```python
from build123d import *

# Parameters (mm, degrees)
BOSS_EXTRUDE1_DEPTH      = 355.6
BOSS_EXTRUDE1_DEPTH_BACK = 254
SKETCH1_R                = 66.04
FILLET1_R                = 12.7
SKETCH3_R                = 12.7
CUT_EXTRUDE1_DEPTH       = 25.4
CHAMFER1_SIZE            = 1.27
FILLET2_R                = 2.54
BOSS_EXTRUDE2_DEPTH      = 600
BOSS_EXTRUDE2_DEPTH_BACK = 583.65
SKETCH4_R                = 120
FILLET3_R                = 20
FILLET4_R                = 90


# Read off the part's stored shape, not the designer's step: Shell1
with BuildPart() as part:
    # Sketch1 → Boss-Extrude1 (new, two sides: drawn at the far end of the back side and taken through both)
    with BuildSketch(Plane.XY.offset(-BOSS_EXTRUDE1_DEPTH_BACK)):
        Circle(SKETCH1_R)
    extrude(amount=BOSS_EXTRUDE1_DEPTH + BOSS_EXTRUDE1_DEPTH_BACK)

    # Sketch2 → Cut-Revolve1 (revolve, cut)
    with BuildSketch(Plane(origin=(0, 0, 0), x_dir=(0, 0, -1), z_dir=(1, 0, 0)), mode=Mode.PRIVATE) as cut_revolve1_sk:
        with BuildLine():
            Line((-355.6, 19.05), (-330.2, 19.05))
            ThreePointArc((-330.2, 19.05), (-306.35774098, 53.006337357), (-266.967262435, 66.04))
            Line((-266.967262435, 66.04), (-355.6, 66.04))
            Line((-355.6, 66.04), (-355.6, 19.05))
        make_face()
    revolve(cut_revolve1_sk.sketch.rotate(Axis((0, 0, 355.6), (0, 0, -1)), 90), axis=Axis((0, 0, 355.6), (0, 0, -1)), mode=Mode.SUBTRACT)

    # Fillet1
    fillet1_edges = [part.edges().sort_by_distance(p)[0] for p in [
        (-66.04, 0, -254),
    ]]
    fillet(fillet1_edges, radius=FILLET1_R)

    # Sketch3 → Cut-Extrude1 (cut)
    with BuildSketch(Plane.XY.offset(355.6)):
        Circle(SKETCH3_R)
    extrude(amount=-CUT_EXTRUDE1_DEPTH, mode=Mode.SUBTRACT)

    # Shell1 outline → Shell1 (revolve, cut)
    with BuildSketch(Plane.XZ):
        with BuildLine():
            Line((0, -247.65), (53.34, -247.65))
            ThreePointArc((53.34, -247.65), (57.830128061, -245.790128061), (59.69, -241.3))
            Line((59.69, -241.3), (59.69, 266.967262375))
            ThreePointArc((59.69, 266.967262375), (46.480959005, 304.416114887), (12.699999942, 325.290551964))
            Line((12.699999942, 325.290551964), (12.7, 330.2))
            Line((12.7, 330.2), (0, 330.2))
            Line((0, 330.2), (0, -247.65))
        make_face()
    revolve(axis=Axis((0, 0, 0), (0, 0, 1)), mode=Mode.SUBTRACT)

    # Chamfer1
    chamfer1_edges = [part.edges().sort_by_distance(p)[0] for p in [
        (-19.05, 0, 355.6),
    ]]
    chamfer(chamfer1_edges, length=CHAMFER1_SIZE)

    # Fillet2
    fillet2_edges = [part.edges().sort_by_distance(p)[0] for p in [
        (-19.05, 0, 330.2),
    ]]
    fillet(fillet2_edges, radius=FILLET2_R)

    # Sketch4 → Boss-Extrude2 (add, two sides: drawn at the far end of the back side and taken through both)
    with BuildSketch(Plane(origin=(0, 0, -254), x_dir=(-1, 0, 0), z_dir=(0, 0, -1)).offset(-BOSS_EXTRUDE2_DEPTH_BACK)):
        Circle(SKETCH4_R)
    extrude(amount=BOSS_EXTRUDE2_DEPTH + BOSS_EXTRUDE2_DEPTH_BACK)

    # Fillet3
    fillet3_edges = [part.edges().sort_by_distance(p)[0] for p in [
        (120, 0, -854),
    ]]
    fillet(fillet3_edges, radius=FILLET3_R)

    # Fillet4
    fillet4_edges = [part.edges().sort_by_distance(p)[0] for p in [
        (120, 0, 329.65),
    ]]
    fillet(fillet4_edges, radius=FILLET4_R)


solid = part.part
```
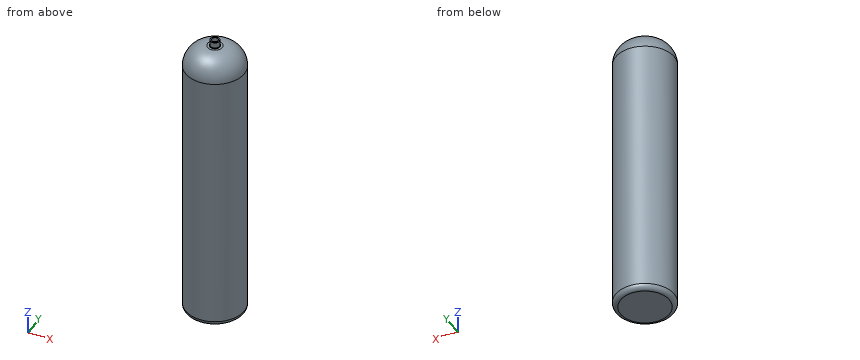
Source: CAD feature listing. Evaluate the final solid. Frame: model axes, mm. Round coordinates to 2 decimals unless told otherwise and drop trailing zeros. Loops run counter-clockwise (first coordinate to the right, second up) from the corner with the lowest first, then second, coordinate; pieces in that order, holes last. Notation, with made-up numbers: M 74,73 L 91,73 A16 cw 91,90 Z; hole C 35.25,-8.5 d9. An arc over 180 degrees is marked long. Use a Markdown table: item, result. Add a question column.
1. Ray query, line 1 along Y through (x, z) = (0, 347.25); line 2 along Z through (x, y) = (40.5, -47.5); line 3 along Z through (x, y) = (-32, 89). Return the intervals inside material, ascending. Write a range as [from, to].
2. Contact query for flat-ended pins moving along their axis: pin 1 (12 mm diameter, centred on y = -69.5, z = -482, fed in from +X); pin 2 (12.5 mm diameter, centred on x = 6, y = -3, fed in from +Z); pin 3 (1 mm diameter, centred on y = -69.5, z = -166.5, fed in from -X); pin 4 (4 mm diameter, centred on x = 75, y = 10, fed in from +Z). Output: stop coordinate, or through.
3. Cut plane A-A, the plane z = -520.5. Output: boundary loops of the cut face in (x, y).
Solution:
| question | item | result |
|---|---|---|
| 1 | line 1 | y = [-19.05, -12.7], [12.7, 19.05] |
| 1 | line 2 | z = [-854, 323.61] |
| 1 | line 3 | z = [-854, 302.34] |
| 2 | pin 1 | stops at x = 101.82 |
| 2 | pin 2 | stops at z = 355.6 |
| 2 | pin 3 | stops at x = -98.18 |
| 2 | pin 4 | stops at z = 318.35 |
| 3 | outline | C 0,0 d240 |
